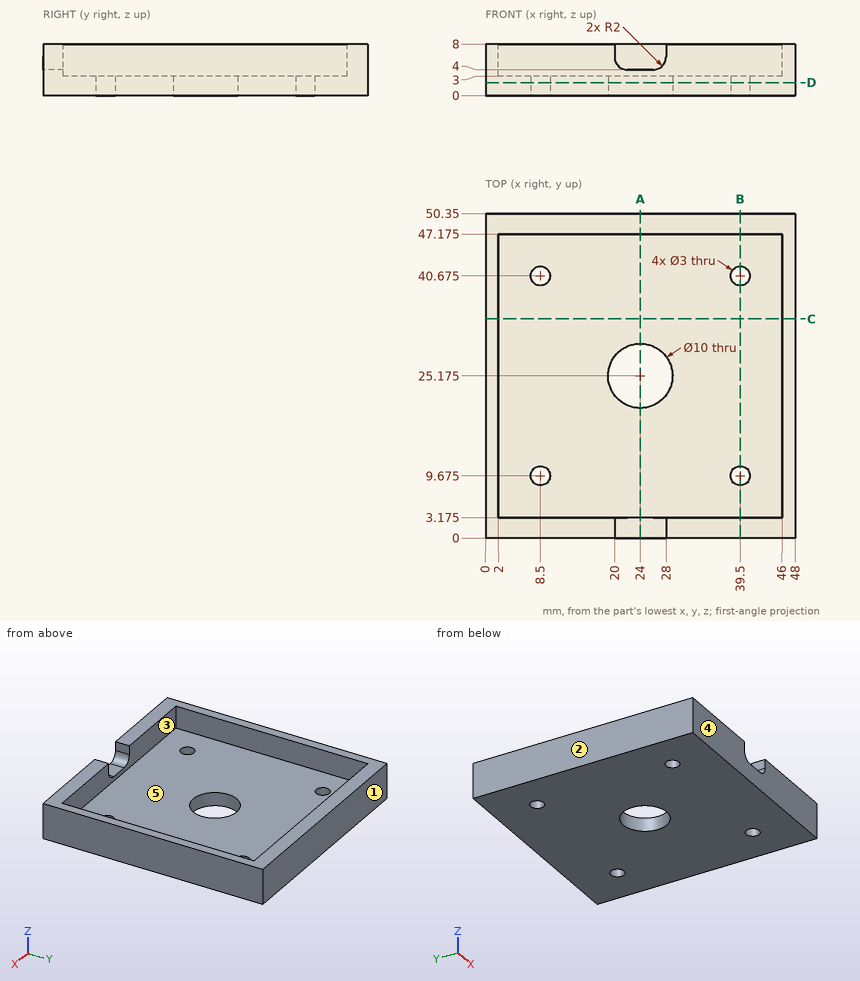
Study the drawing (mm; zero at the part's minimum x, y, z) and answer. A direction names the side the tool comes from. Round coordinates to 2 decimals unless told otherwise and drop trailing zeros. Loops run counter-clockwise (first coordinate to the right, second up) from the corner with the lowest first, then second, coordinate; pieces in that order, holes last. Notation, with made-up numbers: (-37, 3) - (15, 3) arc R23 cw to (15, 36) - close; hole circle Ø9 at (-20, 7). An arc over 180 degrees is marked (long way). Use one line per item in the form item = value. Start each with the question number.
1. Consider line 1 (Y direction, x = 8.5, z = 1.65) (3 decimals); line 2 (X direction, y = 44, z = 5.5); line 3 (Y direction, x = 24, z = 0.65) (3 decimals). Determine where each line is inside the solid, lowest interval first. Write a range as [from, to].
2. The part is cut by section B-B on x = 39.5. Determine the outline of the cut face in (y, z) (3 decimals).
3. The part is cut by section A-A on x = 24. Determine the outline of the cut face in (y, z) (3 decimals).
4. Given pin 1 Ø22 at (x, y) = (34, 16.5) entering from +Z; pin 2 Ø9 at (x, y) = (24, 25.175) entering from -Z; pin 3 Ø1.5 at (x, z) = (24.5, 6) entering from -Y (3 decimals); pin 4 Ø3.5 at (x, y) = (24.5, 2) entering from +Z, each flat-ended and moving along its own axis, determine where each tip first touches the part or whether it passes through.
5. A tool of negligible diameter and unlimited length cuts with its end or side. For the marked faces 4 and 5, from which of +Z, -Z, +X, -X, +Y, -Y can it reach the whole face along a straight path? Write none if from no direction.
6. For a pull along Y with two mould halves and no side action, classify the marked faces 1, 2 and 3 as pulls with the +Y half, pulls with the -Y half, needs draft (parallel to the pull), parting line crosses it, or undercut.
7. The part is cut by section D-D on z = 2. Determine the outline of the cut face in (x, y) (3 decimals), then the cut area to 3 significant figures.
8. The part is cut by section C-C on y = 34. Determine the outline of the cut face in (x, z).
Geometry check:
q1.line_1 = [0, 8.175], [11.175, 39.175], [42.175, 50.35]
q1.line_2 = [0, 2], [46, 48]
q1.line_3 = [0, 20.175], [30.175, 50.35]
q2.outline = (0, 0) - (8.175, 0) - (8.175, 3) - (3.175, 3) - (3.175, 8) - (0, 8) - close; (11.175, 0) - (39.175, 0) - (39.175, 3) - (11.175, 3) - close; (42.175, 0) - (50.35, 0) - (50.35, 8) - (47.175, 8) - (47.175, 3) - (42.175, 3) - close
q3.outline = (0, 0) - (20.175, 0) - (20.175, 3) - (3.175, 3) - (3.175, 4) - (0, 4) - close; (30.175, 0) - (50.35, 0) - (50.35, 8) - (47.175, 8) - (47.175, 3) - (30.175, 3) - close
q4.pin_1 = 3
q4.pin_2 = through
q4.pin_3 = 47.175
q4.pin_4 = 4.02
q5.face_4 = +Z, -Z, +X, -X, -Y
q5.face_5 = +Z
q6.face_1 = pulls with the +Y half
q6.face_2 = needs draft
q6.face_3 = undercut
q7.outline = (0, 0) - (48, 0) - (48, 50.35) - (0, 50.35) - close; hole circle Ø3 at (8.5, 9.675); hole circle Ø3 at (8.5, 40.675); hole circle Ø10 at (24, 25.175); hole circle Ø3 at (39.5, 9.675); hole circle Ø3 at (39.5, 40.675)
q7.area = 2,310 mm^2
q8.outline = (0, 0) - (48, 0) - (48, 8) - (46, 8) - (46, 3) - (2, 3) - (2, 8) - (0, 8) - close
